from build123d import *

# Parameters (mm, degrees)
SKETCH1_W          = 6.879166709
SKETCH1_H          = 3.96875
CUT_EXTRUDE1_DEPTH = 11.506990329
CIRPATTERN1_COUNT  = 24
SKETCH26_W         = 3.571875
SKETCH26_H         = 3.96875
HOLE1_D            = 3.175
SKETCH29_W         = 1.27
SKETCH29_H         = 5.926666709


with BuildPart() as part:
    # Sketch1 → Revolve1 (revolve)
    with BuildSketch(Plane(origin=(0, 0, 0), x_dir=(1, 0, 0), z_dir=(0, 1, 0))):
        with Locations((3.439583355, -1.984375)):
            Rectangle(SKETCH1_W, SKETCH1_H)
    revolve(axis=Axis((0, 0, 0), (0, 0, 1)))

    # Sketch2 → Cut-Extrude1 (cut, through all)
    with BuildSketch(Plane(origin=(0, 0, 0), x_dir=(-1, 0, 0), z_dir=(0, 0, -1))):
        with BuildLine():
            ThreePointArc((4.702545407, 5.020856631), (4.187771356, 5.457609887), (3.632666778, 5.841803376))
            ThreePointArc((3.632666778, 5.841803376), (3.513181537, 5.22234108), (3.313448673, 4.623912268))
            ThreePointArc((3.313448673, 4.623912268), (3.46296478, 4.513023566), (3.608772657, 4.397302205))
            ThreePointArc((3.608772657, 4.397302205), (4.135115832, 4.74511411), (4.702545407, 5.020856631))
        make_face()
    cut_extrude1 = extrude(amount=-CUT_EXTRUDE1_DEPTH, mode=Mode.SUBTRACT)

    # CirPattern1: Cut-Extrude1 ×24 about axis
    cirpattern1_axis = Axis((0, 0, 0), (0, 0, 1))
    for i in range(1, CIRPATTERN1_COUNT):
        add(cut_extrude1.rotate(cirpattern1_axis, i * 360 / CIRPATTERN1_COUNT), mode=Mode.SUBTRACT)

    # Sketch26 → Revolve2 (revolve)
    with BuildSketch(Plane(origin=(0, 0, 0), x_dir=(1, 0, 0), z_dir=(0, 1, 0))):
        with Locations((1.7859375, -5.953125)):
            Rectangle(SKETCH26_W, SKETCH26_H)
    revolve(axis=Axis((0, 0, 3.96875), (0, 0, 1)))

    # Hole1 (through all)
    with Locations(Plane(origin=(0, 0, 0), x_dir=(-1, 0, 0), z_dir=(0, 0, -1))):
        with Locations((0, 0)):
            Hole(HOLE1_D / 2)

    # Sketch29 → M2 Clearance Hole1 (revolve, cut)
    with BuildSketch(Plane(origin=(0.9525, 0, 5.953125), x_dir=(0, 0, 1), z_dir=(0, 1, 0))):
        with Locations((0.635, 2.963333355)):
            Rectangle(SKETCH29_W, SKETCH29_H)
    revolve(axis=Axis((-5.3975, 0, 5.953125), (1, 0, 0)), mode=Mode.SUBTRACT)


solid = part.part
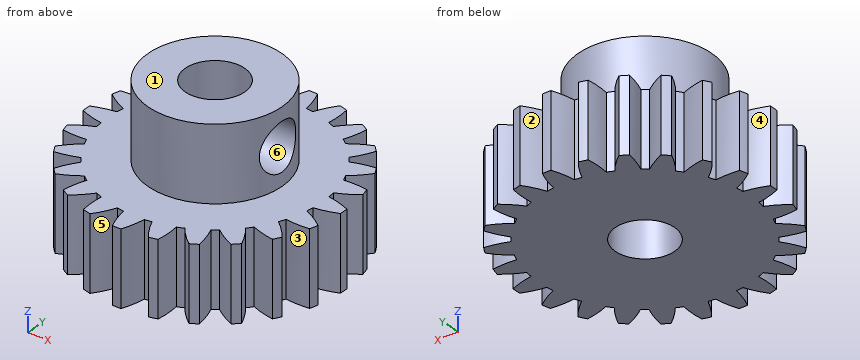
Work out the finished part from the listing and answer in its coordinate system (mm). Face numbers are marked on the shaded views. A direction names the side the tool comes from. Give positions to 0.01 mm unless a question says otherwise; leave off trailing zeros. Loops run counter-clockwise (first coordinate to the right, second up) from the corner with the lowest first, then second, coordinate; pieces in that order, holes last. Notation, with made-up numbers: (32.25, 8) -> (50.25, 8) arc R10 cw to (50.25, 17) -> close; hole circle Ø1 at (68, 68). An arc over 180 degrees is marked (long way). Use a Markdown table: item, result. Add a question column.
1) The part is cut by section C-C, the plane y = 3. Determine the outline of the cut face in (x, z).
2) The part is cut by section B-B, the plane y = 0. Determine the outline of the cut face in (x, z).
3) For a pull along Y with two mould halves and no side action, classify the marked faces 1, 2 and 3 as +Y half, -Y half, draft (parallel to the pull), parting line (faces both ways), or undercut.
4) The part is cut by section A-A, the plane x = 0. Determine the outline of the cut face in (y, z).
5) Consider line 1 along Y through (x, z) = (0, 3.5); line 2 along Z through (x, y) = (2, 0); line 3 along Y through (x, z) = (0, 6.25). Determine where each line is inside the solid, lowest interval first.
6) Which of the six approach directions +Z, -Z, +X, -X, +Y, -Y give full straight-line access (tool end or side, diameter ignored) to the marked faces 4, 5 and 6?
7) This flat-tipped pin is pushed along its axis until it touches: P1, Ø2, axis at x = 0.5, z = 5, coming from the -Y side. Where does it stop, or does it pass through?
Reported:
| question | item | result |
|---|---|---|
| 1 | outline | (-5.87, 0) -> (5.87, 0) -> (5.87, 3.97) -> (1.94, 3.97) -> (1.94, 7.94) -> (-1.94, 7.94) -> (-1.94, 3.97) -> (-5.87, 3.97) -> close |
| 2 | outline | (-6.88, 0) -> (-1.59, 0) -> (-1.59, 7.94) -> (-3.57, 7.94) -> (-3.57, 3.97) -> (-6.88, 3.97) -> close; (1.59, 0) -> (6.88, 0) -> (6.88, 3.97) -> (3.57, 3.97) -> (3.57, 4.68) -> (1.59, 4.68) -> close; (1.59, 7.22) -> (3.57, 7.22) -> (3.57, 7.94) -> (1.59, 7.94) -> close |
| 3 | face 1 | draft |
| 3 | face 2 | +Y half |
| 3 | face 3 | undercut |
| 4 | outline | (-6.88, 0) -> (-1.59, 0) -> (-1.59, 7.94) -> (-3.57, 7.94) -> (-3.57, 3.97) -> (-6.88, 3.97) -> close; (1.59, 0) -> (6.88, 0) -> (6.88, 3.97) -> (3.57, 3.97) -> (3.57, 7.94) -> (1.59, 7.94) -> close |
| 5 | line 1 | y = -6.88 to -1.59, 1.59 to 6.88 |
| 5 | line 2 | z = 0 to 4.68, 7.22 to 7.94 |
| 5 | line 3 | y = -3.57 to -1.59, 1.59 to 3.57 |
| 6 | face 4 | +Z, -Z, -X |
| 6 | face 5 | +Z, -Z, -Y |
| 6 | face 6 | +X |
| 7 | P1 | stops at y = -3.57 |
